Could you check a few things on this model? Use its own coordinates, in mm. A direction names the side the tool comes from. Coordinates: 2 decimals unless noted, no trailing zeros. Write each loop counter-clockwise with the first axis right and the second up, starting at its lowest first coordinate (ties: lowest second). Pieces come first, ordered by that corner, then holes. Notation, with made-up numbers: (5, 5.25) - (11, 5.25) arc R18 cw to (11, 40.25) - close; hole circle Ø7 at (-31, 64.5). An arc over 180 degrees is marked (long way). Answer as a JSON object with one key per item and string values. Group by question number.
1) Please list where these lines run through material, in increasing order: line 1 along Y through (x, z) = (0, 0.6) (3 decimals); line 2 along Z through (x, y) = (8, -1.5); line 3 along X through (y, z) = (0, 0.3) (3 decimals).
2) On a 3-axis mill with a long thin cutter (end or side, diameter ignored), from which of +Z, -Z, +X, -X, +Y, -Y can I reach the whole of each face in a straight line? I mean faces 5 (the flat face through (8.8, 0.9, 0.8)), 6 (the flat face through (4.8, 3.2, 2.5)), 7 (the cylindrical face through (0.629, -4.914, 0.493)), 8 (the flat face through (7, 3, 5)). Say none if no direction works.
3) If we section it at B-B (y = 0): Write out the boundary of the cut face in (x, z) (3 decimals).
4) If we section it at C-C (x = 10.5): Write out the boundary of the cut face in (y, z), plus the area to 3 significant figures.
5) We'd pull the mould along Y, two halves only. Please class faces 1 (the flat face through (5.1, -5.7, 1)), 2 (the cylindrical face through (-0.082, 1.873, 0.493)), 3 (the cylindrical face through (11.29, -11.77, 0.49)), 4 (the cylindrical face through (6.27, -19.88, 0.49)): released by +Y, released by -Y, zero draft, split by the parting line, or undercut.
6) If we section it at D-D (z = 5.75): Write out the boundary of the cut face in (x, y).
7) Will these pins go through, and if not, where does the flat tip stop? pin 1 Ø0.8 at (y, z) = (3.5, 7) entering from +X; pin 2 Ø1.7 at (y, z) = (3, 3) entering from -X; pin 3 Ø12 at (x, y) = (-3, -13) entering from +Z; pin 4 Ø10 at (x, y) = (2.5, -1.5) entering from -Z.
8) If we section it at A-A (x = 0): Write out the boundary of the cut face in (y, z) (3 decimals), plus the area to 3 significant figures.
Autodesk Inventor part; units mm, degrees
ref_plane "YZ Plane" through (0, 0, 0) normal (1, 0, 0) x (0, 1, 0)
ref_plane "XZ Plane" through (0, 0, 0) normal (0, 1, 0) x (-1, 0, 0)
ref_plane "XY Plane" through (0, 0, 0) normal (0, 0, 1) x (1, 0, 0)
sketch "Sketch1 outline for Plate1" plane through (0, 0, 0) normal (0, 0, 1) x (1, 0, 0)
  arc A0 (-4.982963, -20.07059) -> (-4.329627, -20.670078) centre (-4.5, -20.2) ccw
  arc A1 (-4.329627, -20.670078) -> (0.795926, -20.076601) centre (-0.513276, -31.19982) cw
  arc A2 (0.795926, -20.076601) -> (11.300243, -18.119671) centre (2.9, -2.2) ccw
  arc A3 (11.300243, -18.119671) -> (12.481249, -5.626677) centre (7.800142, -11.486475) ccw
  arc A4 (12.481249, -5.626677) -> (8.8, -3.245095) centre (-1.25, -22.815417) ccw
  line L0 (8.8, -3.245095) -> (8.8, 3)
  line L1 (8.8, 3) -> (4.8, 3)
  line L2 (4.8, 3) -> (4.8, 1.83303)
  arc A5 (4.8, 1.83303) -> (3.272727, 1.499752) centre (4, 1.83303) cw
  arc A6 (3.272727, 1.499752) -> (-3.571778, 0.449892) centre (0, 0) ccw
  arc A7 (-3.571778, 0.449892) -> (-5.553237, -1.687388) centre (-6.052179, 0.762317) cw
  arc A8 (-5.553237, -1.687388) -> (-8.642869, -2.560617) centre (-1.25, -22.815417) ccw
  arc A9 (-8.642869, -2.560617) -> (-9.177896, -3.021148) centre (-8.3, -3.5) ccw
  line L3 (-9.177896, -3.021148) -> (-10.377896, -5.221148)
  arc A10 (-10.377896, -5.221148) -> (-9.065789, -6.600811) centre (-9.5, -5.7) ccw
  arc A11 (-9.065789, -6.600811) -> (9.984659, -8.751902) centre (-1.25, -22.815417) cw
  arc A12 (9.984659, -8.751902) -> (9.433522, -14.581966) centre (7.800142, -11.486475) cw
  arc A13 (9.433522, -14.581966) -> (-2.131853, -15.264473) centre (2.9, -2.2) cw
  line L4 (-2.131853, -15.264473) -> (-4.26738, -17.4)
  line L5 (-4.26738, -17.4) -> (-4.982963, -20.07059)
extrude "Plate1" add sketch "Sketch1 outline for Plate1" along normal blind 1
sketch "Sketch2 outline for Plate2" plane through (4.8, 3, 0) normal (0, 1, 0) x (1, 0, 0)
  line L0 (4, -5) -> (4, 0)
  line L1 (3.75, -5) -> (4, -5)
  arc A0 (3.75, -6.5) -> (3.75, -5) centre (3.75, -5.75) cw
  line L2 (4, -6.5) -> (3.75, -6.5)
  line L3 (4, -7.5) -> (4, -6.5)
  line L4 (0, -7.5) -> (4, -7.5)
  line L5 (0, -6.5) -> (0, -7.5)
  line L6 (0.25, -6.5) -> (0, -6.5)
  arc A1 (0.25, -5) -> (0.25, -6.5) centre (0.25, -5.75) cw
  line L7 (0, -5) -> (0.25, -5)
  line L8 (0, 0) -> (0, -5)
  line L9 (4, 0) -> (0, 0)
sheet face with bend "Face2" sketch "Sketch2 outline for Plate2" thickness 1 toward (0, 1, 0) bend radius 1
bend "Bend1"
sketch "Sketch1" plane through (0, 0, 0) normal (0, 0, 1) x (1, 0, 0)
  arc A0 (3.272727, 1.499752) -> (-3.571778, 0.449892) centre (0, 0) ccw
  circle A1 centre (-8.3, -3.5) radius 1
  circle A2 centre (-9.5, -5.7) radius 1
  circle A3 centre (-4.5, -20.2) radius 0.5
  arc A4 (9.984659, -8.751902) -> (-9.065789, -6.600811) centre (-1.25, -22.815417) ccw
  line L0 (0, 0) -> (0, -25.191235) construction
  line L1 (-4.982963, -20.07059) -> (-4.26738, -17.4)
  line L2 (-4.26738, -17.4) -> (-2.131853, -15.264473)
  line L3 (-4.26738, -17.4) -> (1.767607, -17.4) construction
  arc A5 (-2.131853, -15.264473) -> (9.433522, -14.581966) centre (2.9, -2.2) ccw
  arc A6 (9.433522, -14.581966) -> (9.984659, -8.751902) centre (7.800142, -11.486475) ccw
  arc A7 (-5.553237, -1.687388) -> (-8.642869, -2.560617) centre (-1.25, -22.815417) ccw
  arc A8 (0.795926, -20.076601) -> (11.300243, -18.119671) centre (2.9, -2.2) ccw
  arc A9 (11.300243, -18.119671) -> (12.481249, -5.626677) centre (7.800142, -11.486475) ccw
  arc A10 (12.481249, -5.626677) -> (8.8, -3.245095) centre (-1.25, -22.815417) ccw
  line L4 (-10.377896, -5.221148) -> (-9.177896, -3.021148)
  arc A11 (0.795926, -20.076601) -> (-4.329627, -20.670078) centre (-0.513276, -31.19982) ccw
  arc A12 (-5.553237, -1.687388) -> (-3.571778, 0.449892) centre (-6.052179, 0.762317) ccw
  line L5 (4.8, 3) -> (8.8, 3)
  line L6 (8.8, 3) -> (8.8, -3.245095)
  arc A13 (3.272727, 1.499752) -> (4.8, 1.83303) centre (4, 1.83303) ccw
  line L7 (4.8, 3) -> (4.8, 1.83303)
  dimension "d34" = 7.2
  dimension "d35" = 2
  dimension "d36" = 8.3
  dimension "d37" = 9.5
  dimension "d38" = 3.5
  dimension "d39" = 5.7
  dimension "d40" = 1
  dimension "d41" = 20.2
  dimension "d42" = 4.5
  dimension "d43" = 1.25
  dimension "d44" = 22.81542
  dimension "d45" = 18
  dimension "d46" = 15
  dimension "d47" = 17.4
  dimension "d48" = 45
  dimension "d49" = 2.9
  dimension "d50" = 2.2
  dimension "d51" = 14
  dimension "d52" = 3.5
  dimension "d53" = 4
  dimension "d54" = 11.2
  dimension "d55" = 2.5
  dimension "d56" = 8.8
  dimension "d57" = 4
  dimension "d58" = 3
  dimension "d59" = 1.6
  dimension "d60" = 18
  dimension "d61" = 22
sketch "Sketch2" plane through (4.8, 3, 0) normal (0, 1, 0) x (1, 0, 0)
  line L0 (4, 0) -> (0, 0)
  line L1 (4, 0) -> (0, 0)
  line L2 (0, 0) -> (0, -7.5)
  line L3 (0, -7.5) -> (4, -7.5)
  line L4 (4, -7.5) -> (4, 0)
  line L5 (0, -6.5) -> (0.25, -6.5)
  arc A0 (0.25, -6.5) -> (0.25, -5) centre (0.25, -5.75) ccw
  line L6 (0.25, -5) -> (0, -5)
  line L7 (4, -6.5) -> (3.75, -6.5)
  arc A1 (3.75, -5) -> (3.75, -6.5) centre (3.75, -5.75) ccw
  line L8 (3.75, -5) -> (4, -5)
  line L9 (0, -1) -> (4, -1)
  point P0 (-4.8, 0)
  dimension "d65" = 0.75
  dimension "d66" = 3.5
  dimension "d84" = 6.5
  dimension "d85" = 4.75
hole "Hole1" at (0, 0, 1) direction (0, 0, -1) diameter 3.75 end through all
fillet "Fillet1" radius 0.5 2 edges at (-4.2674, -17.4, 0.5) (-2.1319, -15.2645, 0.5)
equation "\"d81\" = Thickness"
equation "\"d86\" = Thickness"
equation "\"d69\" = BendRadius"
equation "\"d70\" = BendReliefWidth"
equation "\"d72\" = MinimumRemnant"
equation "\"d71\" = BendReliefDepth"
equation "\"d73\" = BendRadius"
equation "\"BendRadius\" = Thickness"
equation "\"BendReliefWidth\" = Thickness"
equation "\"BendReliefDepth\" = 0.5 * Thickness"
equation "\"CornerReliefSize\" = 4 * Thickness"
equation "\"MinimumRemnant\" = 2 * Thickness"
equation "\"TransitionRadius\" = BendRadius"
equation "\"JacobiRadiusSize\" = BendRadius"
equation "\"GapSize\" = Thickness"
equation "\"d62\" = BendRadius"
properties part number "403-08" material "Aluminum-6061"
Here are the results:
{
 "1": {"line 1": "y = -20.012 to -15.896, -4.859 to -1.875, 1.875 to 3.6", "line 2": "z = 0 to 1", "line 3": "x = -3.671 to -1.875, 1.875 to 8.8"},
 "2": {"face 5": "+Z, -Z, +X, +Y", "face 6": "+Z, -Z, +Y", "face 7": "+Z, -Z", "face 8": "+Z, +X, -X, -Y"},
 "3": {"outline": "(-3.671, 0) - (-1.875, 0) - (-1.875, 1) - (-3.671, 1) - close; (1.875, 0) - (8.8, 0) - (8.8, 1) - (1.875, 1) - close"},
 "4": {"outline": "(-18.52, 0) - (-13.71, 0) - (-13.71, 1) - (-18.52, 1) - close; (-9.26, 0) - (-4.22, 0) - (-4.22, 1) - (-9.26, 1) - close", "area": "9.85 mm²"},
 "5": {"face 1": "zero draft", "face 2": "undercut", "face 3": "undercut", "face 4": "released by -Y"},
 "6": {"outline": "(5.8, 3) - (7.8, 3) - (7.8, 4) - (5.8, 4) - close"},
 "7": {"pin 1": "stops at x = 8.8", "pin 2": "stops at x = 4.8", "pin 3": "stops at z = 1", "pin 4": "stops at z = 0"},
 "8": {"outline": "(-20.012, 0) - (-15.896, 0) - (-15.896, 1) - (-20.012, 1) - close; (-4.859, 0) - (-1.875, 0) - (-1.875, 1) - (-4.859, 1) - close; (1.875, 0) - (3.6, 0) - (3.6, 1) - (1.875, 1) - close", "area": "8.82 mm²"}
}
